```python
from build123d import *

# Parameters (mm, degrees)
BOSS_EXTRUDE3_DEPTH = 6.35


with BuildPart() as part:
    # Sketch1 → Boss-Extrude3 (new body)
    with BuildSketch(Plane.XY):
        with BuildLine():
            Line((0, 130.023), (0, 143.0035))
            ThreePointArc((0, 143.0035), (-127.347637401, 65.058283566), (-115.871551473, -83.808022119))
            ThreePointArc((-115.871551473, -83.808022119), (-87.648494018, -139.418965385), (-77.925699061, -201.019170265))
            Line((-77.925699061, -201.019170265), (-77.925699061, -225.171))
            Line((-77.925699061, -225.171), (0, -225.171))
            Line((0, -225.171), (0, -130.023))
            ThreePointArc((0, -130.023), (-130.023, 0), (0, 130.023))
        make_face()
    extrude(amount=BOSS_EXTRUDE3_DEPTH)


solid = part.part
```
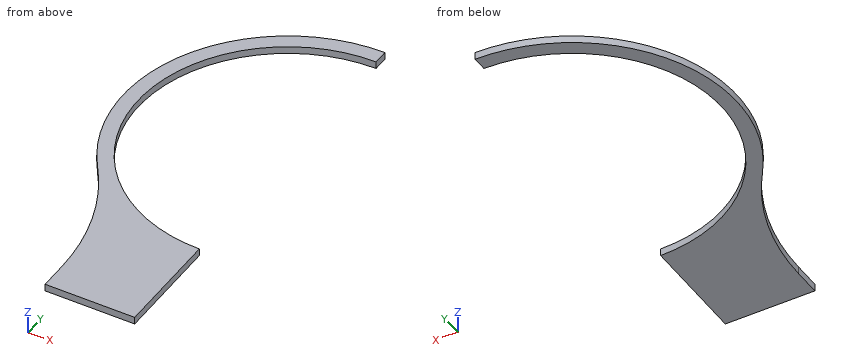
Check sheet for the modelled part. Datum: model origin and axes. Units: mm. Give positions to 0.01 mm unless a question says otherwise; leave off trailing zeros. Order: outer loops, then holes, each group sorted by start corner. A loop starts at its lowest first (then second) coordinate and runs counter-clockwise, first axis right, second up. Notation, with made-up numbers: M 37.25,55.5 L 57.25,55.5 A8 cw 57.25,68.5 Z; hole C 6.25,75.25 d3. An arc over 180 degrees is marked long. Answer in a Markdown table with one row per item. Add a question column.
Q1. Thickness scan on L1, parallel to Y at x = -62, z = 1; L2, parallel to Y at x = -114, z = 5; L3, parallel to X at y = 85, z = 2.5. Record the ranges inside material, lowest first.
Q2. Sectioned sample at C-C, the plane y = 0. Record the boundary of the cut face in (x, z), and give its area (3 significant figures).
Q3. Gauge pin test, flat ends, axial feed: pin 1 Ø2 at (y, z) = (-20.5, 5.5) entering from -X; pin 2 Ø3 at (x, z) = (-126.5, 4) entering from -Y; pin 3 Ø1 at (x, z) = (-83, 1) entering from +Y; pin 4 Ø2 at (y, z) = (-132, 5.5) entering from +X. Record the tip position at first contact, or that the pin passes through.
Q4. Sectioned sample at A-A, the plane z = 2. Record the boundary of the cut face in (x, y), and give its area (3 significant figures).
Q5. Sectioned sample at D-D, the plane x = -21.5. Record the boundary of the cut face in (y, z), and give its area (3 significant figures).
Q6. Sectioned sample at B-B, the plane x = -120. Record the boundary of the cut face in (y, z), and give its area (3 significant figures).
Verdict:
| question | item | result |
|---|---|---|
| 1 | L1 | -225.17 to -114.29, 114.29 to 128.86 |
| 1 | L2 | -86.44 to -62.53, 62.53 to 86.34 |
| 1 | L3 | -115 to -98.39 |
| 2 | outline | M -143,0 L -130.02,0 L -130.02,6.35 L -143,6.35 Z |
| 2 | area | 82.4 mm² |
| 3 | pin 1 | x = -141.67 |
| 3 | pin 2 | y = -69.46 |
| 3 | pin 3 | y = 116.81 |
| 3 | pin 4 | x = 0 |
| 4 | outline | M -115.87,-83.81 A200 cw -77.93,-201.02 L -77.93,-225.17 L 0,-225.17 L 0,-130.02 A130.02 cw 0,130.02 L 0,143 A143 ccw Z |
| 4 | area | 13,200 mm² |
| 5 | outline | M -225.17,0 L -128.23,0 L -128.23,6.35 L -225.17,6.35 Z; M 128.23,0 L 141.38,0 L 141.38,6.35 L 128.23,6.35 Z |
| 5 | area | 699 mm² |
| 6 | outline | M -77.78,0 L -50.06,0 L -50.06,6.35 L -77.78,6.35 Z; M 50.06,0 L 77.78,0 L 77.78,6.35 L 50.06,6.35 Z |
| 6 | area | 352 mm² |
